```python
from build123d import *

# Parameters (mm, degrees)
F0_W      = 73.406
F0_H      = 31.75
F1_DEPTH  = 14.224
F2_W      = 6.35
F2_H      = 28.575
F3_DEPTH  = 7.874
F5_DEPTH  = 7.874
F6_DEPTH  = 3.048
F8_DEPTH  = 4.826
F10_DEPTH = 4.826


with BuildPart() as f1:
    # F0 (on Top) → F1 (new body)
    with BuildSketch(Plane.XY):
        Rectangle(F0_W, F0_H)
    extrude(amount=F1_DEPTH)

    # F2 (on Front) → F3 (join)
    with BuildSketch(Plane.XZ):
        Polygon((-30.353, 42.799), (-30.353, 14.224), (39.37, 14.224), (50.3207743978, 25.1747743978), (32.893, 25.1747743978), (32.893, 42.799), align=None)
        with BuildLine():
            ThreePointArc((-6.4773515256, 22.860703056), (-12.0649999994, 28.4484341748), (-6.4771862369, 34.0360000025))
            Line((-6.4771862369, 34.0360000025), (17.3101380153, 34.035296348))
            ThreePointArc((17.3101380153, 34.035296348), (17.3987768094, 34.0359967795), (17.4874155619, 34.035291104))
            ThreePointArc((17.4874155619, 34.035291104), (22.9864344307, 28.4035107074), (17.3984462114, 22.8599967844))
            Line((17.3984462114, 22.8599967844), (-6.4773515256, 22.860703056))
        make_face(mode=Mode.SUBTRACT)
        Polygon((67.945, 42.799), (32.893, 42.799), (32.893, 25.1747743978), (50.3207743978, 25.1747743978), align=None)
        with Locations((-33.528, 28.5115)):
            Rectangle(F2_W, F2_H)
    extrude(amount=-F3_DEPTH)

    # F4 (on face) → F5 (join)
    with BuildSketch(Plane.XZ):
        Polygon((67.945, 42.799), (-30.353, 42.799), (-30.353, 14.224), (36.703, 14.224), (39.37, 14.224), align=None)
        with BuildLine():
            ThreePointArc((17.3101380153, 34.035296348), (22.9864370529, 28.4921522689), (17.3984462114, 22.8599967844))
            Line((17.3984462114, 22.8599967844), (-6.4773515256, 22.860703056))
            ThreePointArc((-6.4773515256, 22.860703056), (-12.0649999994, 28.4484341748), (-6.4771862369, 34.0360000025))
            Line((-6.4771862369, 34.0360000025), (17.3101380153, 34.035296348))
        make_face(mode=Mode.SUBTRACT)
    extrude(amount=F5_DEPTH)

    # F6 (add): a face of the model
    f6_faces = [f1.faces().sort_by_distance(p)[0] for p in [
        (-33.528, 0, 28.5115),
    ]]
    extrude(f6_faces, amount=F6_DEPTH)

    # F7 (on face) → F8 (join)
    with BuildSketch(Plane.XZ.offset(7.874)):
        Polygon((50.419, 25.273), (67.945, 42.799), (32.893, 42.799), (32.893, 25.273), align=None)
    extrude(amount=F8_DEPTH)

    # F9 (on face) → F10 (join)
    with BuildSketch(Plane(origin=(0, 7.874, 0), x_dir=(-1, 0, 0), z_dir=(0, 1, 0))):
        Polygon((-32.893, 42.799), (-67.945, 42.799), (-50.419, 25.273), (-32.893, 25.273), align=None)
    extrude(amount=F10_DEPTH)

    # F11: F1 across plane


with BuildPart() as f1_1:
    add(f1.part)
    add(f1.part.mirror(Plane.XY))


solid = f1_1.part
```
Geometry: final body of the model. Coordinates: model frame, mm. A direction names the side the tool comes from. Round coordinates to 2 decimals unless told otherwise and drop trailing zeros. Write each loop counter-clockwise with the first axis right and the second up, starting at its lowest first coordinate (ties: lowest second). Pieces come first, ordered by that corner, then holes. Notation, with made-up numbers: (79, 22.25) -> (113, 22.25) arc R7 ccw to (113, 34.25) -> close; hole circle Ø1 at (47, 52.5). An arc over 180 degrees is marked (long way). Return JSON: item names as keys, results as strings.
Q1. Mould query, pull axis Z, two halves, no side actions, for faces 5 (the flat face through (27, 0, 42.799)), 6 (the flat face through (-30.353, -5, 29)), 7 (the flat face through (42, 10, -25.273)). Classes: +Z half, -Z half, draft (parallel to the pull), parting line (faces both ways), or undercut.
From the geometry:
{"face 5": "+Z half", "face 6": "draft", "face 7": "undercut"}
Q2. Section B-B on x = -23. Return the cut outline in (y, z) (3 decimals), and give its area (3 significant figures).
From the geometry:
{"outline": "(-15.875, -14.224) -> (-7.874, -14.224) -> (-7.874, -42.799) -> (7.874, -42.799) -> (7.874, -14.224) -> (15.875, -14.224) -> (15.875, 14.224) -> (7.874, 14.224) -> (7.874, 42.799) -> (-7.874, 42.799) -> (-7.874, 14.224) -> (-15.875, 14.224) -> close", "area": "1,800 mm2"}
Q3. Section A-A on x = 56. Return the cut outline in (y, z).
From the geometry:
{"outline": "(-12.7, -42.8) -> (12.7, -42.8) -> (12.7, -30.85) -> (-12.7, -30.85) -> close; (-12.7, 30.85) -> (12.7, 30.85) -> (12.7, 42.8) -> (-12.7, 42.8) -> close"}
Q4. First-contact query: pin 1 Ø10 at (y, z) = (-11.5, 15.5) entering from +X; pin 2 Ø2.5 at (y, z) = (-5.5, -28) entering from -X; pin 3 Ø8.5 at (x, z) = (-4.5, -31.5) entering from -Y. Flat tips, straight axial feed; report the tip coordinate or a pass-through.
From the geometry:
{"pin 1": "x = 44.09", "pin 2": "x = -30.35", "pin 3": "y = -7.87"}
Q5. Section D-D on x = 8.5. Return the cut outline in (y, z) (3 decimals).
From the geometry:
{"outline": "(-15.875, -14.224) -> (-7.874, -14.224) -> (-7.874, -22.86) -> (7.874, -22.86) -> (7.874, -14.224) -> (15.875, -14.224) -> (15.875, 14.224) -> (7.874, 14.224) -> (7.874, 22.86) -> (-7.874, 22.86) -> (-7.874, 14.224) -> (-15.875, 14.224) -> close; (-7.874, -42.799) -> (7.874, -42.799) -> (7.874, -34.036) -> (-7.874, -34.036) -> close; (-7.874, 34.036) -> (7.874, 34.036) -> (7.874, 42.799) -> (-7.874, 42.799) -> close"}
Q6. Ray query, line 1 (Z direction, x = 9.5, y = -6.5); line 2 (Z direction, x = 36, y = 10.5); line 3 (Z direction, x = -26.5, y = -13). Return the intervals inside material, ascending.
From the geometry:
{"line 1": "-42.8 to -34.04, -22.86 to 22.86, 34.04 to 42.8", "line 2": "-42.8 to -25.27, -14.22 to 14.22, 25.27 to 42.8", "line 3": "-14.22 to 14.22"}
Q7. Section C-C on z = 32.5. Return the cut outline in (x, y), and give its area (3 significant figures).
From the geometry:
{"outline": "(-36.7, -3.05) -> (-30.35, -3.05) -> (-30.35, -7.87) -> (-10.33, -7.87) -> (-10.33, 7.87) -> (-36.7, 7.87) -> close; (21.25, -7.87) -> (32.89, -7.87) -> (32.89, -12.7) -> (57.65, -12.7) -> (57.65, 12.7) -> (32.89, 12.7) -> (32.89, 7.87) -> (21.25, 7.87) -> close", "area": "1,200 mm2"}
Q8. Set-up query: faces 1 (the flat face through (42, 10, 25.273)), 2 (the flat face through (46, -12.7, 34)), 3 (the flat face through (36.703, 0, 0)), 4 (the flat face through (32.893, -10, -34)). Return all of +Z, -Z, +X, -X, +Y, -Y with unobstructed straight access to the full face (end or side cutting, diameter ignored); none if empty.
From the geometry:
{"face 1": "+X, -X, +Y", "face 2": "+Z, +X, -X, -Y", "face 3": "+X, +Y, -Y", "face 4": "-Z, -X, -Y"}
